from build123d import *

# Parameters (mm, degrees)
PLAT_W                      = 60
PLAT_H                      = 15
EL_MENT_M_CANO_SOUD_1_DEPTH = 170
ESQUISSE2_R                 = 7.5
ENL_V_MAT_EXTRU_1_DEPTH     = 16


with BuildPart() as part:
    # plat → Elément mécano-soudé1 (new body)
    with BuildSketch(Plane.YZ.offset(-85)):
        Rectangle(PLAT_W, PLAT_H)
    extrude(amount=EL_MENT_M_CANO_SOUD_1_DEPTH)

    # Esquisse2 → Enlèv. mat.-Extru.1 (cut, through all)
    with BuildSketch(Plane.XY.offset(7.5)):
        with Locations((-15, -8.979692736)):
            Circle(ESQUISSE2_R)
        with Locations((-44.077931835, -1.599050475)):
            Circle(ESQUISSE2_R)
        with Locations((-70.446339823, 12.708537029)):
            Circle(ESQUISSE2_R)
        with Locations(Location((70.446339823, 12.708537029, 0), (0, 0, 180))):  # turned: the seam where the file's is
            Circle(ESQUISSE2_R)
        with Locations(Location((44.077931835, -1.599050475, 0), (0, 0, 180))):  # turned: the seam where the file's is
            Circle(ESQUISSE2_R)
        with Locations(Location((15, -8.979692736, 0), (0, 0, 180))):  # turned: the seam where the file's is
            Circle(ESQUISSE2_R)
    extrude(amount=-ENL_V_MAT_EXTRU_1_DEPTH, mode=Mode.SUBTRACT)


solid = part.part
Check sheet for the modelled part. Datum: model origin and axes. Units: mm. Round coordinates to 2 decimals unless told otherwise and drop trailing zeros. Loops run counter-clockwise (first coordinate to the right, second up) from the corner with the lowest first, then second, coordinate; pieces in that order, holes last. Notation, with made-up numbers: M -20,-21.5 L 31,-21.5 A17 cw 31,-14.5 Z; hole C 2.5,0.25 d5. An arc over 180 degrees is marked long. One line per question, with ' | ' between items. Start each with the question number.
Item 1: Section check D-D (y = -5.5). Record the boundary of the cut face in (x, z).
Item 2: Section check B-B (x = -15). Record the boundary of the cut face in (y, z).
Item 3: Section check A-A (y = -12.5). Record the boundary of the cut face in (x, z).
Item 4: Scan lines: probe 1 along X at (y, z) = (3.5, -3.5); probe 2 along X at (y, z) = (11.5, 0); probe 3 along X at (y, z) = (-4.5, -5.5). Record each from-to range of solid material in increasing order.
Item 5: Section check C-C (z = 1.75). Record the boundary of the cut face in (x, y).
Item 6: Release check for a two-part mould opening along X. For faces 1 (the face through (-85, 0, 0)), 2 (the face through (-1, 0, 7.5)), 3 (the face through (-66.986, 6.055, 0.105)), 4 (the face through (85, 0, 0)) record: released by +X, released by -X, zero draft, split by the parting line, or undercut.
Item 7: Gauge pin test, flat end, axial feed: pin 1 Ø12 at (x, y) = (44.08, -1.6) entering from -Z. Record the tip position at first contact, or that the pin passes through.
Worked out:
1) outline: M -85,-7.5 L -50.48,-7.5 L -50.48,7.5 L -85,7.5 Z; M -37.67,-7.5 L -21.64,-7.5 L -21.64,7.5 L -37.67,7.5 Z; M -8.36,-7.5 L 8.36,-7.5 L 8.36,7.5 L -8.36,7.5 Z; M 21.64,-7.5 L 37.67,-7.5 L 37.67,7.5 L 21.64,7.5 Z; M 50.48,-7.5 L 85,-7.5 L 85,7.5 L 50.48,7.5 Z
2) outline: M -30,-7.5 L -16.48,-7.5 L -16.48,7.5 L -30,7.5 Z; M -1.48,-7.5 L 30,-7.5 L 30,7.5 L -1.48,7.5 Z
3) outline: M -85,-7.5 L -21.62,-7.5 L -21.62,7.5 L -85,7.5 Z; M -8.38,-7.5 L 8.38,-7.5 L 8.38,7.5 L -8.38,7.5 Z; M 21.62,-7.5 L 85,-7.5 L 85,7.5 L 21.62,7.5 Z
4) probe 1: -85 to -49.58, -38.58 to 38.58, 49.58 to 85 | probe 2: -85 to -77.85, -63.04 to 63.04, 77.85 to 85 | probe 3: -85 to -50.99, -37.16 to -21.02, -8.98 to 8.98, 21.02 to 37.16, 50.99 to 85
5) outline: M -85,-30 L 85,-30 L 85,30 L -85,30 Z; hole C -70.45,12.71 d15; hole C -44.08,-1.6 d15; hole C -15,-8.98 d15; hole C 15,-8.98 d15; hole C 44.08,-1.6 d15; hole C 70.45,12.71 d15
6) face 1: released by -X | face 2: zero draft | face 3: undercut | face 4: released by +X
7) pin 1: through
